Check sheet for the modelled part. Datum: model origin and axes. Units: mm. Coordinates: 2 decimals unless noted, no trailing zeros. Order: outer loops, then holes, each group sorted by start corner. A loop starts at its lowest first (then second) coordinate and runs counter-clockwise, first axis right, second up.
1. Thickness scan on line 1 (X direction, y = -0.5, z = 112); line 2 (Y direction, x = -1.5, z = 14). Record the ranges inside material, lowest first.
2. Gauge pin test, flat ends, axial feed: pin 1 Ø4 at (x, z) = (1, 33.5) entering from -Y; pin 2 Ø2 at (y, z) = (-3.5, 21) entering from +X; pin 3 Ø3 at (y, z) = (3.5, 97.5) entering from -X. Record the tip position at first contact, or that the pin passes through.
3. Cross-section at A-A (z = 130.5). Enter the section's corners in (x, y), then the cut area to 3 significant figures.
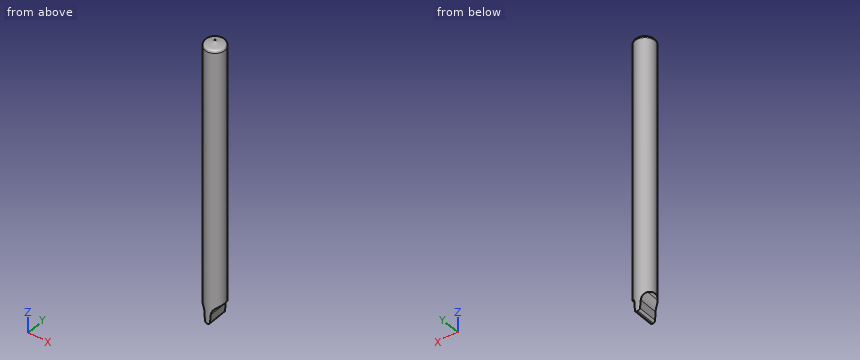
```python
from build123d import *

# Parameters (mm, degrees)
F0_R     = 5
F1_DEPTH = 140
F3_DEPTH = 11.55


with BuildPart() as f1:
    # F0 (on Top) → F1 (new body)
    with BuildSketch(Plane.XY):
        Circle(F0_R)
    extrude(amount=F1_DEPTH)

    # F2 (on Front) → F3 (cut, symmetric)
    with BuildSketch(Plane.XZ):
        with BuildLine():
            ThreePointArc((-4.9343728731, 9.5041744104), (-4.9905112474, 9.5740316018), (-4.9936231851, 9.6635964393))
            Line((-4.9936231851, 9.6635964393), (-5.6447708048, 8.8026849553))
            Line((-5.6447708048, 8.8026849553), (-7.4423355982, 9.3325031921))
            Line((-7.4423355982, 9.3325031921), (-10.4406764731, 4.5940310123))
            Line((-10.4406764731, 4.5940310123), (-9.1289039701, -1.7381435225))
            Line((-9.1289039701, -1.7381435225), (0, -1.7381435225))
            Line((0, -1.7381435225), (8.475315288, -1.7381435225))
            Line((8.475315288, -1.7381435225), (6.0502169654, 5.5752913468))
            Line((6.0502169654, 5.5752913468), (5.1431669854, 9.3325031921))
            Line((5.1431669854, 9.3325031921), (4.9936231851, 9.6635964393))
            ThreePointArc((4.9936231851, 9.6635964393), (4.9905112474, 9.5740316018), (4.9343728731, 9.5041744104))
            Line((4.9343728731, 9.5041744104), (3.8363389221, 8.7961034203))
            ThreePointArc((3.8363389221, 8.7961034203), (2.2446684706, 7.1431548318), (1.5589835431, 4.9532940959))
            Line((1.5589835431, 4.9532940959), (1.2690167304, 0.9281473833))
            ThreePointArc((1.2690167304, 0.9281473833), (0.9528310141, 0.2679301206), (0.2716014701, 0))
            Line((0.2716014701, 0), (0, 0))
            Line((0, 0), (-0.2716014701, 0))
            ThreePointArc((-0.2716014701, 0), (-0.9528310141, 0.2679301206), (-1.2690167304, 0.9281473833))
            Line((-1.2690167304, 0.9281473833), (-1.5589835431, 4.9532940959))
            ThreePointArc((-1.5589835431, 4.9532940959), (-2.2446684706, 7.1431548318), (-3.8363389221, 8.7961034203))
            Line((-3.8363389221, 8.7961034203), (-4.9343728731, 9.5041744104))
        make_face()
    extrude(amount=F3_DEPTH, both=True, mode=Mode.SUBTRACT)

    # F4 (on Right) → F5 (revolve, cut)
    with BuildSketch(Plane.YZ):
        with BuildLine():
            Line((-0.0064786935, 140.206694603), (-5.0473981754, 140.206694603))
            Line((-5.0473981754, 140.206694603), (-5.0473981754, 136.6430294396))
            add(Edge.make_bspline(
                [(-0.0064786935, 140.0043070316), (-0.0692082586, 139.9860955088), (-0.1979467492, 139.9487204058), (-0.2136150513, 139.7256958309), (-0.2745325567, 139.409206263), (-0.3981966452, 138.9202736287), (-3.584305469, 138.5722227649), (-4.3554143689, 138.43019256), (-4.7752856256, 137.9991725277), (-4.916967026, 137.7419277902), (-4.9952783408, 137.0821454066), (-5.0473981754, 136.6430294396)],
                knots=[0, 0, 0, 0, 0.0599452364, 0.1230242745, 0.2025770079, 0.2903198787, 0.5396616387, 0.6742796245, 0.7743510294, 0.8498200795, 1, 1, 1, 1], degree=3))
            Line((-0.0064786935, 140.0043070316), (-0.0064786935, 140.206694603))
        make_face()
    revolve(axis=Axis((0, 0, 139.283709228), (0, 0, -1)), mode=Mode.SUBTRACT)


solid = f1.part
```
Data:
1. line 1: x = -4.97 to 4.97
1. line 2: y = -4.77 to 4.77
2. pin 1: stops at y = -5
2. pin 2: stops at x = 4.33
2. pin 3: stops at x = -4.58
3. outline: circle Ø10 at (0, 0)
3. area: 78.5 mm2
